```python
from build123d import *

# Parameters (mm, degrees)
SKETCH1_R           = 18
BOSS_EXTRUDE1_DEPTH = 58
SKETCH2_R           = 1.5875
BOSS_EXTRUDE2_DEPTH = 16.5
SKETCH3_R           = 1.5
CUT_EXTRUDE1_DEPTH  = 5
SKETCH3_3_R         = 6.5
SKETCH3_3_R_2       = 1.5875
BOSS_EXTRUDE3_DEPTH = 4.5


with BuildPart() as part:
    # Sketch1 → Boss-Extrude1 (new body)
    with BuildSketch(Plane(origin=(0, 0, 0), x_dir=(1, 0, 0), z_dir=(0, 1, 0))):
        Circle(SKETCH1_R)
    extrude(amount=BOSS_EXTRUDE1_DEPTH)

    # Sketch2 → Boss-Extrude2 (add)
    with BuildSketch(Plane.XZ):
        Circle(SKETCH2_R)
    extrude(amount=BOSS_EXTRUDE2_DEPTH)

    # Sketch3 → Cut-Extrude1 (cut)
    with BuildSketch(Plane(origin=(0, 0, 0), x_dir=(-1, 0, 0), z_dir=(0, -1, 0))):
        with Locations((-12.5, 0)):
            Circle(SKETCH3_R)
        with Locations((12.5, 0)):
            Circle(SKETCH3_R)
    extrude(amount=-CUT_EXTRUDE1_DEPTH, mode=Mode.SUBTRACT)

    # Sketch3<3> → Boss-Extrude3 (add)
    with BuildSketch(Plane(origin=(0, 0, 0), x_dir=(-1, 0, 0), z_dir=(0, -1, 0))):
        Circle(SKETCH3_3_R)
        Circle(SKETCH3_3_R_2, mode=Mode.SUBTRACT)
    extrude(amount=BOSS_EXTRUDE3_DEPTH)


solid = part.part
```
Build history of the part. All positions in model axes, mm. A direction names the side the tool comes from. Round coordinates to 2 decimals unless told otherwise and drop trailing zeros. Write each loop counter-clockwise with the first axis right and the second up, starting at its lowest first coordinate (ties: lowest second). Pieces come first, ordered by that corner, then holes. Notation, with made-up numbers: (-8.5, 62.5) - (12.5, 62.5) arc R29 ccw to (12.5, 83.5) - close; hole circle Ø2 at (-39.75, 88). An arc over 180 degrees is marked (long way). Write each question's results on one line, items separated by ' | '. Start each with the question number.
Item 1: Saw through at C-C (y = -9). Write the cut outline in (x, z) (1 decimal), and give its area (3 significant figures).
Item 2: Wall check: L1, parallel to X at y = 1, z = 0; L2, parallel to Y at x = -2, z = 5.5; L3, parallel to Y at x = 9, z = -11.5. Give the ranges that are in metal, low to high. Write a range as [from, to].
Item 3: Saw through at D-D (x = -12.5). Write the cut outline in (y, z), and give its area (3 significant figures).
Item 4: Which spindle directions (+Z, -Z, +X, -X, +Y, -Y) get a long thin tool onto all of the face, cutting with end or side? Do faces 1 (the face through (0, 0, 8)), 2 (the face through (-2.343, 28.594, -17.847)). Say none if no direction does.
Item 5: Saw through at B-B (z = 0). Write the cut outline in (x, y), and give its area (3 significant figures).
Item 6: Drop flat-ended pins along their axis: P1, Ø5, axis at x = 4, z = 6, coming from the -Y side; P2, Ø6.5, axis at x = 2, z = 1, coming from the -Y side; P3, Ø1.5, axis at x = -12, z = -0.5, coming from the -Y side; P4, Ø3, axis at x = 2, y = 6, coming from the +Z side. Give the stop position or say it passes through.
Item 7: Mould opens along X. For faces 3 (the face through (14, 2, 0)), 4 (the face through (-1.4, -4.5, 1.4)), 5 (the face through (-0.34, -10.42, -1.55)) say: pulls with the +X half, pulls with the -X half, needs draft (parallel to the pull), parting line crosses it, or undercut.
Item 8: Saw through at A-A (x = 0). Write the cut outline in (y, z), and give its area (3 significant figures).
Results are:
1) outline: circle Ø3.2 at (0, 0) | area: 7.92 mm²
2) L1: x = [-18, -14], [-11, 11], [14, 18] | L2: y = [-4.5, 58] | L3: y = [0, 58]
3) outline: (0, -12.95) - (58, -12.95) - (58, 12.95) - (0, 12.95) - (0, 1.5) - (5, 1.5) - (5, -1.5) - (0, -1.5) - close | area: 1,490 mm²
4) face 1: -Y | face 2: +Y, -Y
5) outline: (-18, 0) - (-14, 0) - (-14, 5) - (-11, 5) - (-11, 0) - (-6.5, 0) - (-6.5, -4.5) - (-1.59, -4.5) - (-1.59, -16.5) - (1.59, -16.5) - (1.59, -4.5) - (6.5, -4.5) - (6.5, 0) - (11, 0) - (11, 5) - (14, 5) - (14, 0) - (18, 0) - (18, 58) - (-18, 58) - close | area: 2,150 mm²
6) P1: stops at y = -4.5 | P2: stops at y = -16.5 | P3: stops at y = 5 | P4: stops at z = 17.99
7) face 3: undercut | face 4: needs draft | face 5: parting line crosses it
8) outline: (-16.5, -1.59) - (-4.5, -1.59) - (-4.5, -6.5) - (0, -6.5) - (0, -18) - (58, -18) - (58, 18) - (0, 18) - (0, 6.5) - (-4.5, 6.5) - (-4.5, 1.59) - (-16.5, 1.59) - close | area: 2,180 mm²
